For this review, take the finished solid that the model builds, in its own axes (mm). A direction names the side the tool comes from. Coordinates: 2 decimals unless noted, no trailing zeros. Order: outer loops, then holes, each group sorted by start corner. A loop starts at its lowest first (then second) coordinate and runs counter-clockwise, first axis right, second up. Notation, with made-up numbers: M -30.75,-23.5 L 9.25,-23.5 A22 ccw 9.25,9.5 Z; hole C 51.25,34 d10. An arc over 180 degrees is marked long. Use CSV: the item, a comma, the result in double quotes.
```python
from build123d import *

# Parameters (mm, degrees)
SKETCH1_W           = 36.58
SKETCH1_H           = 20
SKETCH1_R           = 1.25
BOSS_EXTRUDE1_DEPTH = 5
SKETCH3_W           = 20
SKETCH3_H           = 30
SKETCH3_W_2         = 10
SKETCH3_H_2         = 41
BOSS_EXTRUDE2_DEPTH = 7
FILLET1_R           = 3
FILLET2_R           = 1
CUT_EXTRUDE1_REACH  = 101.795
SKETCH6_R           = 1.4
FILLET3_R           = 2


with BuildPart() as part:
    # Sketch1 → Boss-Extrude1 (new body)
    with BuildSketch(Plane(origin=(0, 0, 0), x_dir=(1, 0, 0), z_dir=(0, 1, 0))):
        with Locations((18.29, 10)):
            Rectangle(SKETCH1_W, SKETCH1_H)
        with Locations(Location((25.58, 3, 0), (0, 0, 270))):
            Circle(SKETCH1_R, mode=Mode.SUBTRACT)
        with Locations(Location((33.58, 3, 0), (0, 0, 270))):
            Circle(SKETCH1_R, mode=Mode.SUBTRACT)
        with Locations(Location((33.58, 17, 0), (0, 0, 90))):
            Circle(SKETCH1_R, mode=Mode.SUBTRACT)
        with Locations(Location((25.58, 17, 0), (0, 0, 90))):
            Circle(SKETCH1_R, mode=Mode.SUBTRACT)
    extrude(amount=BOSS_EXTRUDE1_DEPTH)

    # Sketch3 → Boss-Extrude2 (add)
    with BuildSketch(Plane.ZY):
        with Locations((-10, 20)):
            Rectangle(SKETCH3_W, SKETCH3_H)
        Polygon((-20, 20), (-20, 35), (-25, 35), (-30, 35), align=None)
        with Locations((-30, 55.5)):
            Rectangle(SKETCH3_W_2, SKETCH3_H_2)
        Polygon((-25, 76), (5, 76), (15, 76), (15, 86), (-35, 86), (-35, 76), align=None)
        with Locations((10, 55.5)):
            Rectangle(SKETCH3_W_2, SKETCH3_H_2)
        Polygon((5, 35), (0, 35), (0, 20), (10, 35), align=None)
    extrude(amount=-BOSS_EXTRUDE2_DEPTH)

    # Fillet1
    fillet1_edges = [part.edges().sort_by_distance(p)[0] for p in [
        (3.5, 86, 15),
        (3.5, 35, 15),
        (3.5, 35, -35),
        (3.5, 86, -35),
    ]]
    fillet(fillet1_edges, radius=FILLET1_R)

    # Fillet2
    fillet2_edges = [part.edges().sort_by_distance(p)[0] for p in [
        (3.5, 35, 10),
        (3.5, 35, -30),
    ]]
    fillet(fillet2_edges, radius=FILLET2_R)

    # Sketch6 → Cut-Extrude1 (cut, up to next)
    with BuildSketch(Plane.ZY, mode=Mode.PRIVATE) as cut_extrude1_sk1:
        with Locations((-15, 31.5)):
            Circle(SKETCH6_R)
    cut_extrude1_tool1 = extrude(cut_extrude1_sk1.sketch, amount=-CUT_EXTRUDE1_REACH, mode=Mode.PRIVATE) & part.part
    # Sketch6 → Cut-Extrude1 (cut, up to next)
    with BuildSketch(Plane.ZY, mode=Mode.PRIVATE) as cut_extrude1_sk2:
        with Locations((-5, 31.5)):
            Circle(SKETCH6_R)
    cut_extrude1_tool2 = extrude(cut_extrude1_sk2.sketch, amount=-CUT_EXTRUDE1_REACH, mode=Mode.PRIVATE) & part.part
    # Sketch6 → Cut-Extrude1 (cut, up to next)
    with BuildSketch(Plane.ZY, mode=Mode.PRIVATE) as cut_extrude1_sk3:
        with Locations((-15, 79.5)):
            Circle(SKETCH6_R)
    cut_extrude1_tool3 = extrude(cut_extrude1_sk3.sketch, amount=-CUT_EXTRUDE1_REACH, mode=Mode.PRIVATE) & part.part
    # Sketch6 → Cut-Extrude1 (cut, up to next)
    with BuildSketch(Plane.ZY, mode=Mode.PRIVATE) as cut_extrude1_sk4:
        with Locations((-5, 79.5)):
            Circle(SKETCH6_R)
    cut_extrude1_tool4 = extrude(cut_extrude1_sk4.sketch, amount=-CUT_EXTRUDE1_REACH, mode=Mode.PRIVATE) & part.part
    add(cut_extrude1_tool1.solids().sort_by_distance((0, 31.5, -15))[0], mode=Mode.SUBTRACT)
    add(cut_extrude1_tool2.solids().sort_by_distance((0, 31.5, -5))[0], mode=Mode.SUBTRACT)
    add(cut_extrude1_tool3.solids().sort_by_distance((0, 79.5, -15))[0], mode=Mode.SUBTRACT)
    add(cut_extrude1_tool4.solids().sort_by_distance((0, 79.5, -5))[0], mode=Mode.SUBTRACT)

    # Fillet3
    fillet3_edges = [part.edges().sort_by_distance(p)[0] for p in [
        (3.5, 76, 5),
        (3.5, 76, -25),
        (3.5, 35, -25),
        (3.5, 35, 5),
        (7, 5, -10),
    ]]
    fillet(fillet3_edges, radius=FILLET3_R)


solid = part.part
```
Item 1: Add section B-B on x = 4. State the section outline as (y, z) points, and give its area (3 significant figures).
Solutions:
outline,"M 0,-20 L 20,-20 L 34.55,-29.7 A1 cw 35,-30.54 L 35,-32 A3 ccw 38,-35 L 83,-35 A3 ccw 86,-32 L 86,12 A3 ccw 83,15 L 38,15 A3 ccw 35,12 L 35,10.54 A1 cw 34.55,9.7 L 20,0 L 0,0 Z; hole C 31.5,-15 d2.8; hole C 31.5,-5 d2.8; hole M 35,-23 A2 ccw 37,-25 L 74,-25 A2 ccw 76,-23 L 76,3 A2 ccw 74,5 L 37,5 A2 ccw 35,3 Z; hole C 79.5,-15 d2.8; hole C 79.5,-5 d2.8"
area,"2,140 mm^2"
Item 2: For faces 5 (the face through (10, 3, 0)), 6 (the face through (3, 55, 5)), 7 (the face through (36.58, 2, -10)), 8 (the face through (10, 3, -20)), list the 3-axis set-ups (+Z, -Z, +X, -X, +Y, -Y) from which the entire face can be reached by the end or side of a thin tool; tool diameter is ignored.
Solutions:
face 5,"+Z, +X, -X, -Y"
face 6,"+X, -X"
face 7,"+Z, -Z, +X, +Y, -Y"
face 8,"-Z, +X, -X, -Y"
Item 3: Add section D-D on y = 29. State the section outline as (x, z) points, and give its area (3 significant figures).
Solutions:
outline,"M 0,-26 L 7,-26 L 7,6 L 0,6 Z"
area,"224 mm^2"
Item 4: Add section A-A on y = 53. State the section outline as (x, z) points.
Solutions:
outline,"M 0,-35 L 7,-35 L 7,-25 L 0,-25 Z; M 0,5 L 7,5 L 7,15 L 0,15 Z"
Item 5: To check wall thickness, follow line 1 along Z through (x, y) = (4.5, 79.5); line 2 along Y through (x, z) = (3, -5); line 3 along X through (y, z) = (1.6, -3). State the ranges of each line that lie inside material, in increasing order. Write a range as [from, to].
Solutions:
line 1,"[-35, -16.4], [-13.6, -6.4], [-3.6, 15]"
line 2,"[0, 30.1], [32.9, 35], [76, 78.1], [80.9, 86]"
line 3,"[0, 24.33], [26.83, 32.33], [34.83, 36.58]"
Item 6: Clearance check with flat-ended pins moving along their axes: pin 1 Ø1.2 at (x, z) = (4.5, 11) entering from -Y; pin 2 Ø2 at (x, z) = (33.58, -17) entering from -Y; pin 3 Ø16 at (x, y) = (12.5, 11) entering from -Z. State where each tip first meets the part, or that it passes through.
Solutions:
pin 1,"y = 34.99"
pin 2,"through"
pin 3,"z = -20"
Item 7: Draft analysis for pull direction Y (two halves, no side actions). For faces 1 (the face through (3.55, 75.4, -24.43)), 2 (the face through (3.55, 35.9, 14.14)), 3 (the face through (32.471, 2.465, -2.423)), 4 (the face through (23, 5, -10)), state which applies: released by +Y, released by -Y, zero draft, split by the parting line, or undercut.
Solutions:
face 1,"undercut"
face 2,"released by -Y"
face 3,"zero draft"
face 4,"released by +Y"
Item 8: Add section C-C on x = 21.5. State the section outline as (y, z) points.
Solutions:
outline,"M 0,-20 L 5,-20 L 5,0 L 0,0 Z"
